Verification items for the finished model (mm, model axes). Face numbers are marked on the shaded views. A direction names the side the tool comes from. Give positions to 0.01 mm unless a question says otherwise; leave off trailing zeros. Order: outer loops, then holes, each group sorted by start corner. A loop starts at its lowest first (then second) coordinate and runs counter-clockwise, first axis right, second up.
from build123d import *

# Parameters (mm, degrees)
F0_W     = 120.65
F0_H     = 120.65
F1_DEPTH = 139.7
F2_T     = -5.08
F4_DEPTH = 25.4
F5_R     = 1.5875
F6_DEPTH = 25.4


with BuildPart() as f1:
    # F0 (on Top) → F1 (new body)
    with BuildSketch(Plane.XY):
        with Locations((-21.288729769, 17.728820008)):
            Rectangle(F0_W, F0_H)
    extrude(amount=F1_DEPTH)

    # F2
    f2_openings = [f1.faces().sort_by_distance(p)[0] for p in [
        (-21.28873, 17.72882, 139.7),
    ]]
    offset(amount=F2_T, openings=f2_openings)

    # F3 (on face) → F4 (cut)
    with BuildSketch(Plane(origin=(-81.613729769, 0, 0), x_dir=(0, -1, 0), z_dir=(-1, 0, 0))):
        with BuildLine():
            Line((-22.8087121331, 79.4233293937), (-22.8087121331, 129.9203726467))
            ThreePointArc((-22.8087121331, 129.9203726467), (-27.9420685988, 129.1377325739), (-32.9687117108, 127.8351454898))
            Line((-32.9687117108, 127.8351454898), (-32.9687117108, 79.4203999617))
            Line((-32.9687117108, 79.4203999617), (-22.8087121331, 79.4233293937))
        make_face()
        with BuildLine():
            ThreePointArc((-32.9687117108, 30.9148545102), (-27.9420685988, 29.6122674261), (-22.8087121331, 28.8296273533))
            Line((-22.8087121331, 28.8296273533), (-22.8087121331, 79.4233293937))
            Line((-22.8087121331, 79.4233293937), (-32.9687117108, 79.4203999617))
            Line((-32.9687117108, 79.4203999617), (-32.9687117108, 30.9148545102))
        make_face()
        with BuildLine():
            ThreePointArc((-12.6196735848, 28.8325760096), (-7.486767718, 29.618187754), (-2.4608762974, 30.9236853135))
            Line((-2.4608762974, 30.9236853135), (-2.4748441512, 79.3676804493))
            Line((-2.4748441512, 79.3676804493), (-2.4888187622, 79.36767642))
            Line((-2.4888187622, 79.36767642), (-12.6342468971, 79.3764521102))
            Line((-12.6342468971, 79.3764521102), (-12.6196735848, 28.8325760096))
        make_face()
        with BuildLine():
            Line((-2.4748441512, 79.3676804493), (-2.4888187622, 127.8351110402))
            ThreePointArc((-2.4888187622, 127.8351110402), (-7.5154621752, 129.1377101531), (-12.6488202192, 129.9203618262))
            Line((-12.6488202192, 129.9203618262), (-12.6342468971, 79.3764521102))
            Line((-12.6342468971, 79.3764521102), (-2.4888187622, 79.36767642))
            Line((-2.4888187622, 79.36767642), (-2.4748441512, 79.3676804493))
        make_face()
        with BuildLine():
            Line((17.8416409794, 79.3735383001), (17.8311803932, 115.6534560237))
            ThreePointArc((17.8311803932, 115.6534560237), (12.9943502285, 119.8314804526), (7.6711808155, 123.3690900368))
            Line((7.6711808155, 123.3690900368), (7.6711808155, 79.370605852))
            Line((7.6711808155, 79.370605852), (17.8311803932, 79.373535284))
            Line((17.8311803932, 79.373535284), (17.8416409794, 79.3735383001))
        make_face()
        with BuildLine():
            ThreePointArc((7.6711808155, 35.3809099632), (13.0060137652, 38.9273796382), (17.8520948084, 43.1170560315))
            Line((17.8520948084, 43.1170560315), (17.8416409794, 79.3735383001))
            Line((17.8416409794, 79.3735383001), (17.8311803932, 79.373535284))
            Line((17.8311803932, 79.373535284), (7.6711808155, 79.370605852))
            Line((7.6711808155, 79.370605852), (7.6711808155, 35.3809099632))
        make_face()
        with BuildLine():
            Line((27.9975640978, 79.376464716), (33.0711799708, 79.376464716))
            ThreePointArc((33.0711799708, 79.376464716), (31.7847314928, 90.7349391624), (27.9911799708, 101.5182066768))
            Line((27.9911799708, 101.5182066768), (27.9975640978, 79.376464716))
        make_face()
        with BuildLine():
            ThreePointArc((28.0039414666, 57.2581618917), (31.7881684046, 68.0300514084), (33.071179992, 79.375))
            ThreePointArc((33.071179992, 79.375), (33.0711799867, 79.375732358), (33.0711799708, 79.376464716))
            Line((33.0711799708, 79.376464716), (27.9975640978, 79.376464716))
            Line((27.9975640978, 79.376464716), (28.0039414666, 57.2581618917))
        make_face()
        with BuildLine():
            Line((-42.9323247395, 79.4203999617), (-43.1287117108, 123.3691530375))
            ThreePointArc((-43.1287117108, 123.3691530375), (-48.4518229046, 119.8316075323), (-53.2886102754, 115.6536619949))
            Line((-53.2886102754, 115.6536619949), (-53.1265006866, 79.375724394))
            Line((-53.1265006866, 79.375724394), (-43.1287117108, 79.4203999617))
            Line((-43.1287117108, 79.4203999617), (-42.9323247395, 79.4203999617))
        make_face()
        with BuildLine():
            ThreePointArc((-52.962971018, 42.7799921081), (-48.0890388763, 38.6454393558), (-42.7345255311, 35.155607294))
            Line((-42.7345255311, 35.155607294), (-42.9323247395, 79.4203999617))
            Line((-42.9323247395, 79.4203999617), (-43.1287117108, 79.4203999617))
            Line((-43.1287117108, 79.4203999617), (-53.1265006866, 79.375724394))
            Line((-53.1265006866, 79.375724394), (-52.962971018, 42.7799921081))
        make_face()
        with BuildLine():
            Line((-63.4422243346, 79.3720724091), (-63.4486098531, 101.5186405436))
            ThreePointArc((-63.4486098531, 101.5186405436), (-67.2429726273, 90.732318803), (-68.528819818, 79.3706057914))
            Line((-68.528819818, 79.3706057914), (-63.4486098531, 79.372070568))
            Line((-63.4486098531, 79.372070568), (-63.4422243346, 79.3720724091))
        make_face()
        with BuildLine():
            ThreePointArc((-68.528819818, 79.3706057914), (-67.2387120843, 67.9991226008), (-63.4358329036, 57.2049983725))
            Line((-63.4358329036, 57.2049983725), (-63.4422243346, 79.3720724091))
            Line((-63.4422243346, 79.3720724091), (-63.4486098531, 79.372070568))
            Line((-63.4486098531, 79.372070568), (-68.528819818, 79.3706057914))
        make_face()
    extrude(amount=-F4_DEPTH, mode=Mode.SUBTRACT)

    # F5 (on face) → F6 (cut)
    with BuildSketch(Plane(origin=(-81.613729769, 0, 0), x_dir=(0, -1, 0), z_dir=(-1, 0, 0))):
        with Locations((34.6613678069, 27.1940474238)):
            Circle(F5_R)
        with Locations((-70.0808512879, 131.7625792464)):
            Circle(F5_R)
    extrude(amount=-F6_DEPTH, mode=Mode.SUBTRACT)


solid = f1.part
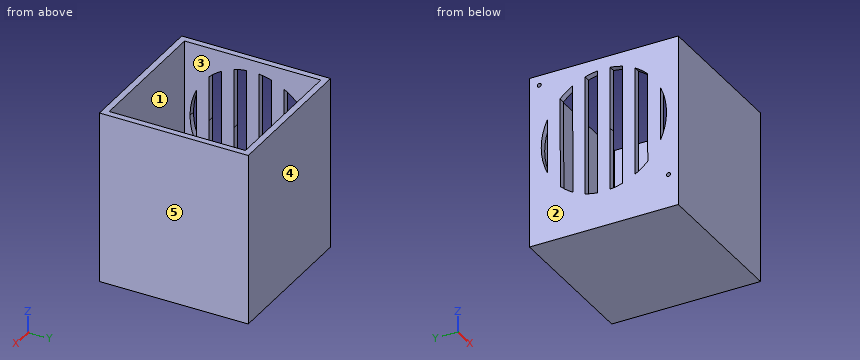
(1) Section check D-D, the plane x = -59.5. Enter the section's corners in (y, z), then the cut area to 3 significant figures.
Solved:
outline: (-42.6, 0) - (78.05, 0) - (78.05, 139.7) - (72.97, 139.7) - (72.97, 5.08) - (-37.52, 5.08) - (-37.52, 139.7) - (-42.6, 139.7) - close
area: 1,980 mm2
(2) Section check B-B, the plane y = 27.5. Enter the section's corners in (x, z), then the cut area to 3 significant figures.
Solved:
outline: (-81.61, 0) - (39.04, 0) - (39.04, 139.7) - (33.96, 139.7) - (33.96, 5.08) - (-76.53, 5.08) - (-76.53, 29.52) - (-81.61, 29.52) - close; (-81.61, 129.23) - (-76.53, 129.23) - (-76.53, 139.7) - (-81.61, 139.7) - close
area: 1,470 mm2
(3) Release check for a two-part mould opening along X. For the marked faces 3, 4 and 5 record: pulls with the +X half, pulls with the -X half, needs draft (parallel to the pull), parting line crosses it, or undercut.
Solved:
face 3: undercut
face 4: needs draft
face 5: pulls with the +X half
(4) Set-up check for the marked faces 1 and 2: record each of +Z, -Z, +X, -X, +Y, -Y from which the full face is reachable in a straight line by a thin tool's end or side.
Solved:
face 1: +Z
face 2: +Z, -Z, -X, +Y, -Y
(5) Scan lines: line 1 (Y direction, x = -46, z = 68); line 2 (X direction, y = -33, z = 132); line 3 (Z direction, x = -54, y = -21.5). Record each from-to range of solid material in increasing order.
Solved:
line 1: y = -42.6 to -37.52, 72.97 to 78.05
line 2: x = -81.61 to -76.53, 33.96 to 39.04
line 3: z = 0 to 5.08
(6) Go/stop test with flat-tipped pins: pin 1 (12 mm diameter, centred on x = -49.5, y = -7, fed in from +Z); pin 2 (8 mm diameter, centred on x = 9.5, y = 54, fed in from -Z). Record where each tip stops, or that it passes through.
Solved:
pin 1: stops at z = 5.08
pin 2: stops at z = 0
(7) Section check C-C, the plane z = 119. Enter the section's corners in (x, y).
Solved:
outline: (-81.61, -42.6) - (39.04, -42.6) - (39.04, 78.05) - (-81.61, 78.05) - (-81.61, 49.52) - (-76.53, 49.52) - (-76.53, 72.97) - (33.96, 72.97) - (33.96, -37.52) - (-76.53, -37.52) - (-76.53, -14.06) - (-81.61, -14.06) - close; (-81.61, -7.67) - (-76.53, -7.67) - (-76.53, 2.49) - (-81.61, 2.49) - close; (-81.61, 12.65) - (-76.53, 12.65) - (-76.53, 22.81) - (-81.61, 22.81) - close; (-81.61, 32.97) - (-76.53, 32.97) - (-76.53, 43.11) - (-81.61, 43.11) - close
(8) Section check A-A, the plane z = 92.5. Give the number of separate pieces and of enclosed holes in the cut face, then the cut area to 3 significant figures.
Solved:
separate pieces: 6
enclosed holes: 0
area: 2,110 mm2
